from build123d import *

# Parameters (mm, degrees)
SKETCH_1_W      = 100
SKETCH_1_H      = 100
EXTRUDE_1_DEPTH = 3
SKETCH_1_3_W    = 100
SKETCH_1_3_H    = 100
SKETCH_1_3_W_2  = 94
SKETCH_1_3_H_2  = 94
EXTRUDE_2_DEPTH = 90


with BuildPart() as part:
    # 草图1 → 凸台-拉伸1 (new body)
    with BuildSketch(Plane(origin=(0, 0, 0), x_dir=(1, 0, 0), z_dir=(0, 1, 0))):
        with Locations((50, -50)):
            Rectangle(SKETCH_1_W, SKETCH_1_H)
    extrude(amount=EXTRUDE_1_DEPTH)

    # 草图1<3> → 凸台-拉伸2 (add)
    with BuildSketch(Plane(origin=(0, 0, 0), x_dir=(1, 0, 0), z_dir=(0, 1, 0))):
        with Locations((50, -50)):
            Rectangle(SKETCH_1_3_W, SKETCH_1_3_H)
        with Locations((50, -50)):
            Rectangle(SKETCH_1_3_W_2, SKETCH_1_3_H_2, mode=Mode.SUBTRACT)
    extrude(amount=-EXTRUDE_2_DEPTH)


solid = part.part
Geometry check sheet. Reference: the model listing, model coordinates, mm. A direction names the side the tool comes from. Give positions to 0.01 mm unless a question says otherwise; leave off trailing zeros. Loops run counter-clockwise (first coordinate to the right, second up) from the corner with the lowest first, then second, coordinate; pieces in that order, holes last. Notation, with made-up numbers: M 2.25,-40 L 23.25,-40 A24 cw 23.25,-26 Z; hole C -19,67 d8. An arc over 180 degrees is marked long. Answer as a JSON object with one key per item and string values. Group by question number.
Item 1: Sectioned sample at B-B on y = -55. Record the boundary of the cut face in (x, z).
Item 2: Mould release check, pull along X, two halves, no side actions. Record for faces 3 (the flat face through (49, 0, 49)), 4 (the flat face through (0, -43, 51)), 5 (the flat face through (49, -43, 100)): pulls with the +X half, pulls with the -X half, needs draft (parallel to the pull), parting line crosses it, or undercut.
Item 3: Sectioned sample at C-C on x = 22. Record the boundary of the cut face in (y, z).
Item 4: Sectioned sample at A-A on z = 27. Record the boundary of the cut face in (x, y).
Item 5: Access from +Z, -Z, +X, -X, +Y, -Y to the whole of each face (thin tool, end or side, straight path). Record for faces 1 (the flat face through (100, -43, 51)), 2 (the flat face through (3, -44, 51)).
Item 6: Material ranges on L1, parallel to Z at x = 54.5, y = -39.5; L2, parallel to Y at x = 64, z = 92, recorded low to high.
Item 7: Gauge pin test, flat end, axial feed: pin 1 (8 mm diameter, centred on x = 47.5, z = 76, fed in from -Y). Record the tip position at first contact, or that the pin passes through.
Findings below:
{
 "1": {"outline": "M 0,0 L 100,0 L 100,100 L 0,100 Z; hole M 3,3 L 97,3 L 97,97 L 3,97 Z"},
 "2": {"face 3": "undercut", "face 4": "pulls with the -X half", "face 5": "needs draft"},
 "3": {"outline": "M -90,0 L 3,0 L 3,100 L -90,100 L -90,97 L 0,97 L 0,3 L -90,3 Z"},
 "4": {"outline": "M 0,-90 L 3,-90 L 3,0 L 97,0 L 97,-90 L 100,-90 L 100,3 L 0,3 Z"},
 "5": {"face 1": "+Z, -Z, +X, +Y, -Y", "face 2": "-Y"},
 "6": {"L1": "0 to 3, 97 to 100", "L2": "0 to 3"},
 "7": {"pin 1": "y = 0"}
}
